Part print with two shaded views. Sizes in mm from the minimum x, y, z corner. A direction names the side the tool comes from. Coordinates: 2 decimals unless noted, no trailing zeros. Loops run counter-clockwise (first coordinate to the right, second up) from the corner with the lowest first, then second, coordinate; pieces in that order, holes last.
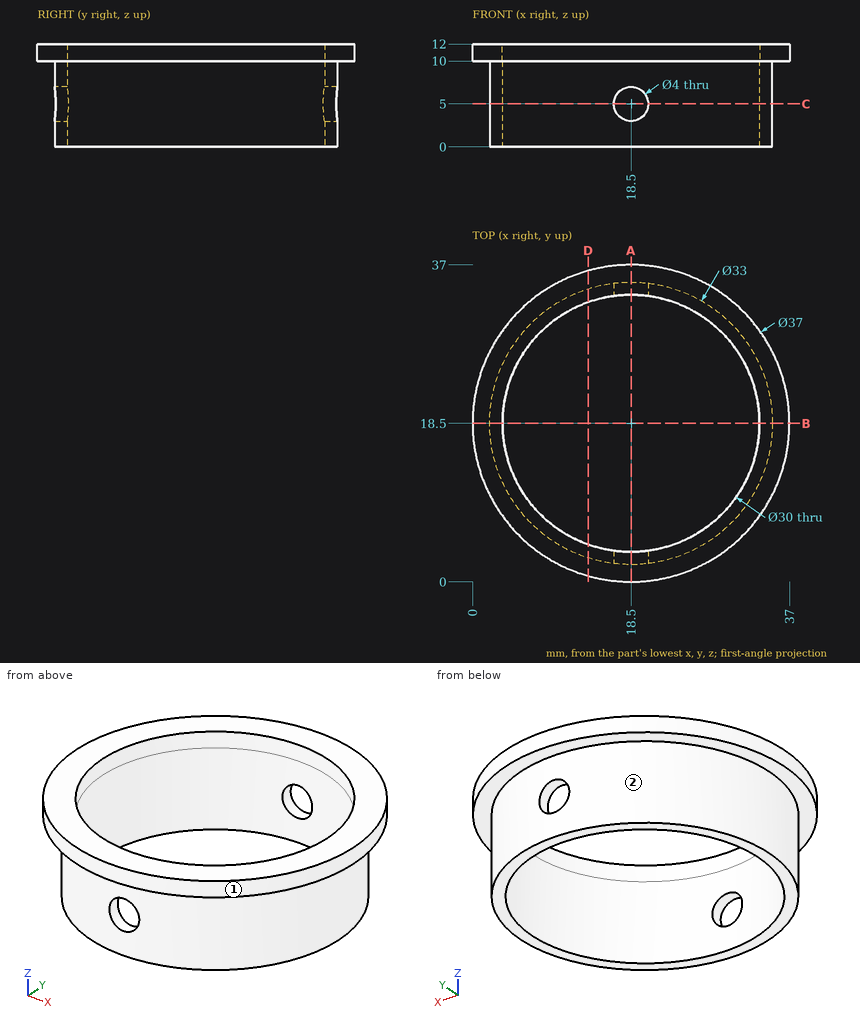
Q1. Which spindle directions (+Z, -Z, +X, -X, +Y, -Y) get a long thin tool onto all of the face, cutting with end or side? Do the marked faces 1 and 2. Say none if no direction does.
Answers:
face 1: +Z, -Z
face 2: -Z
Q2. Slice it at D-D (x = 13.5). List the corners of the cut face in (y, z).
Answers:
outline: (0.69, 10) - (2.78, 10) - (2.78, 0) - (4.36, 0) - (4.36, 12) - (0.69, 12) - close; (32.64, 0) - (34.22, 0) - (34.22, 10) - (36.31, 10) - (36.31, 12) - (32.64, 12) - close
Q3. Slice it at C-C (z = 5). List the corners of the cut face in (x, y), and give its area (3 significant figures).
Answers:
outline: (16.5, 2.12) - (16.5, 3.63) arc R15 cw to (16.5, 33.37) - (16.5, 34.88) arc R16.5 ccw to start; (20.5, 2.12) arc R16.5 ccw to (20.5, 34.88) - (20.5, 33.37) arc R15 cw to (20.5, 3.63) - close
area: 136 mm2
Q4. Slice it at B-B (y = 18.5). List the corners of the cut face in (x, z), and give its area (3 significant figures).
Answers:
outline: (0, 10) - (2, 10) - (2, 0) - (3.5, 0) - (3.5, 12) - (0, 12) - close; (33.5, 0) - (35, 0) - (35, 10) - (37, 10) - (37, 12) - (33.5, 12) - close
area: 44.0 mm2
Q5. Flat gauge pins, fed straight in: P1, Ø5, axis at x = 18.5, z = 5, coming from the +Y side; P2, Ø3, axis at y = 9.5, z = 3.5, coming from the -X side; P3, Ø1, axis at x = 9.5, z = 2, coming from the -Y side; P4, Ø4, axis at x = 20.5, y = 29.5, coming from the +Z side. Where does each tip first touch, or does it go through?
Answers:
P1: stops at y = 35
P2: stops at x = 3.8
P3: stops at y = 4.36
P4: passes through
Q6. Slice it at A-A (x = 18.5). List the corners of the cut face in (y, z), and give its area (3 significant figures).
Answers:
outline: (0, 10) - (2, 10) - (2, 7) - (3.5, 7) - (3.5, 12) - (0, 12) - close; (2, 0) - (3.5, 0) - (3.5, 3) - (2, 3) - close; (33.5, 0) - (35, 0) - (35, 3) - (33.5, 3) - close; (33.5, 7) - (35, 7) - (35, 10) - (37, 10) - (37, 12) - (33.5, 12) - close
area: 32.0 mm2
Q7. Drill centre lines: line 1 (Y direction, x = 18.5, z = 11.05); line 2 (X direction, y = 18.5, z = 3.25); line 3 (Z direction, x = 18.5, y = 2.45). Where is each one in solid material? Low to high.
Answers:
line 1: y = 0 to 3.5, 33.5 to 37
line 2: x = 2 to 3.5, 33.5 to 35
line 3: z = 0 to 3, 7 to 12
